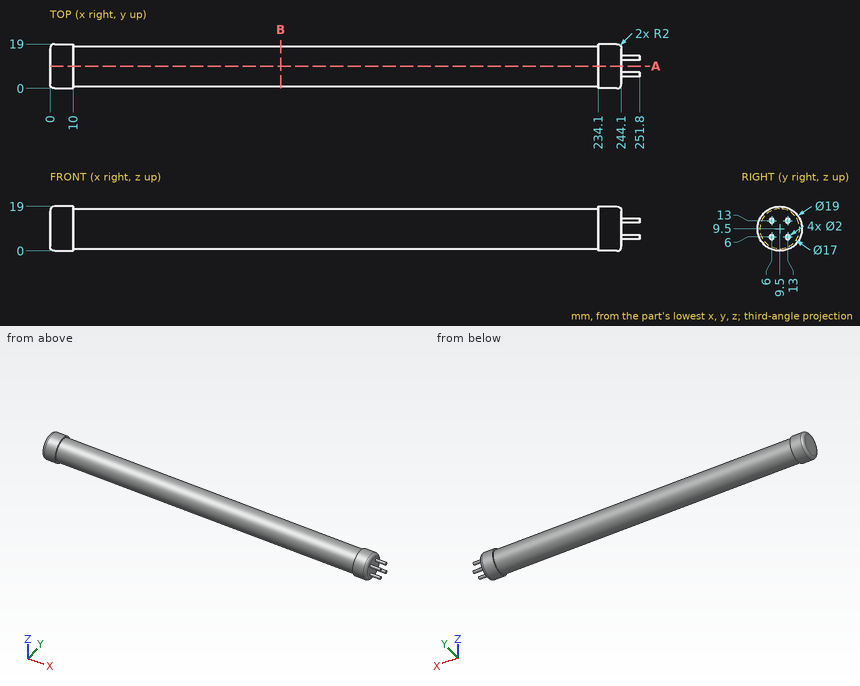
Print and shaded views of the part. All mm, measured from the part's lowest x, y and z. Round coordinates to 2 decimals unless told otherwise and drop trailing zeros. Write each loop counter-clockwise with the first axis right and the second up, starting at its lowest first coordinate (ties: lowest second). Pieces come first, ordered by that corner, then holes. Notation, with made-up numbers: (-35, 6) - (-16, 6) arc R28 ccw to (-16, 38) - close; hole circle Ø6 at (39, 87.5). An arc over 180 degrees is marked (long way). Use CSV: the item, a comma, the result in double quotes. Start each with the question number.
Item 1: Pin check, flat tips, straight feed: P1, Ø1.5, axis at y = 6, z = 9, coming from the +X side; P2, Ø4, axis at x = 57.5, z = 9.5, coming from the +Y side; P3, Ø3, axis at x = 92, z = 12, coming from the +Y side. Stop position of each tip, or through.
Item 2: Drill centre lines: L1, parallel to X at y = 6.5, z = 15.25; L2, parallel to Y at x = 236, z = 9; L3, parallel to Y at x = 179.5, z = 9.75. Where is each one in solid material? Low to high. Write a range as [from, to].
Item 3: Band-saw the part on B-B (x = 98.5). Write the cut outline in (y, z), and give its area (3 significant figures).
Item 4: Band-saw the part on A-A (y = 9.5). Write the cut outline in (x, z).
Checked values:
1,P1,"stops at x = 244.1"
1,P2,"stops at y = 18"
1,P3,"stops at y = 17.94"
2,L1,"x = [0, 244.1]"
2,L2,"y = [0.01, 18.99]"
2,L3,"y = [1, 18]"
3,outline,"circle Ø17 at (9.5, 9.5)"
3,area,"227 mm²"
4,outline,"(0, 2) arc R2 ccw to (2, 0) - (10, 0) - (10, 1) - (234.1, 1) - (234.1, 0) - (242.1, 0) arc R2 ccw to (244.1, 2) - (244.1, 17) arc R2 ccw to (242.1, 19) - (234.1, 19) - (234.1, 18) - (10, 18) - (10, 19) - (2, 19) arc R2 ccw to (0, 17) - close"
